Read the model definition and answer for the solid it produces. Units are mm, in the model's axes. Face numbers are marked on the shaded views. A direction names the side the tool comes from. Give positions to 0.01 mm unless a question says otherwise; leave off trailing zeros. Loops run counter-clockwise (first coordinate to the right, second up) from the corner with the lowest first, then second, coordinate; pieces in that order, holes last.
(1) Each of these flat-tipped pins is pushed along its axis until it touches: P1, Ø4, axis at y = 20.5, z = 24.5, coming from the +X side; P2, Ø5, axis at x = 26.5, y = 12, coming from the +Z side; P3, Ø2, axis at x = 18.5, z = 6.5, coming from the +Y side. Where does it stop, or does it pass through?
(2) Determine the mould class of the marked faces 6, 7, 8 and 9 for opening direction Z: pulls with the +Z half, pulls with the -Z half, needs draft (parallel to the pull), parting line crosses it, or undercut.
(3) Which of the six approach directions +Z, -Z, +X, -X, +Y, -Y give full straight-line access (tool end or side, diameter ignored) to the marked faces 1, 2, 3, 4 and 5?
(4) Find section D-D, the plane z = 13. Write down the section's boundary in (x, y), then the cut area to 3 significant figures.
(5) Find section A-A, the plane z = 6. Write down the section's boundary in (x, y), then the cut area to 3 significant figures.
(6) Find section B-B, the plane y = 41.5. Write down the section's boundary in (x, z).
(7) Find section C-C, the plane y = 22.5. Write down the section's boundary in (x, z).
(8) Straight lines are drawn through the part: probe 1 along Y at (x, z) = (19, 9); probe 2 along X at (y, z) = (35, 3.75); probe 3 along Y at (x, z) = (19.2, 12.25). For each, find the intervals that lie inside material, in ascending order.
```python
from build123d import *

# Parameters (mm, degrees)
F1_DEPTH       = 25
F2_W           = 15
F2_H           = 15
F3_DEPTH       = 45
F4_R           = 2
F6_D           = 4
F8_D           = 4
F8_DEPTH       = 15
F8_CSINK_D     = 4.5
F8_CSINK_ANGLE = 90
F8_TIP         = 1.2017212381
F9_R           = 2
F10_DEPTH      = 45
F11_W          = 13.5859974714
F11_H          = 15
F12_DEPTH      = 25.4


with BuildPart() as f1:
    # F0 (on Right) → F1 (new body)
    with BuildSketch(Plane.YZ):
        Polygon((0, 4), (0, 0), (45, 0), (45, 4), (39.5, 4), (39.5, 11), (45, 11), (45, 34), (0, 34), (0, 11), (5.5, 11), (5.5, 4), align=None)
    extrude(amount=F1_DEPTH)

    # F2 (on face) → F3 (cut, through all)
    with BuildSketch(Plane.XZ):
        with Locations((17.5, 26.5)):
            Rectangle(F2_W, F2_H)
    extrude(amount=-F3_DEPTH, mode=Mode.SUBTRACT)

    # F4
    f4_edges = [f1.edges().sort_by_distance(p)[0] for p in [
        (10, 22.5, 34),
        (5, 0, 34),
        (5, 45, 34),
    ]]
    fillet(f4_edges, radius=F4_R)

    # F6 (through all)
    with Locations(Plane(origin=(0, 0, 0), x_dir=(0, -1, 0), z_dir=(-1, 0, 0))):
        with Locations((-22.5, 6)):
            Hole(F6_D / 2)

    # F8
    with Locations(Plane(origin=(0, 0, 0), x_dir=(1, 0, 0), z_dir=(0, 0, -1))):
        with Locations((19.2, -9.6), (6.5, -9.6), (6.5, -35), (19.2, -35)):
            CounterSinkHole(F8_D / 2, F8_CSINK_D / 2, depth=F8_DEPTH, counter_sink_angle=F8_CSINK_ANGLE)
            with Locations((0, 0, -(F8_DEPTH + F8_TIP / 2))):  # 118° drill point
                Cone(0, F8_D / 2, F8_TIP, mode=Mode.SUBTRACT)

    # F9 (on face) → F10 (join, through all)
    with BuildSketch(Plane.XZ):
        with BuildLine():
            Line((32, 19), (25, 19))
            Line((25, 19), (25, 11))
            Line((25, 11), (25.65, 11))
            ThreePointArc((25.65, 11), (30.1401280605, 12.8598719395), (32, 17.35))
            Line((32, 17.35), (32, 19))
        make_face()
        with Locations((28.9811789989, 16.233060509)):
            Circle(F9_R, mode=Mode.SUBTRACT)
    extrude(amount=-F10_DEPTH)

    # F11 (on face) → F12 (cut)
    with BuildSketch(Plane(origin=(0, 0, 0), x_dir=(1, 0, 0), z_dir=(0, 0, -1))):
        with Locations((31.7929987357, -22.5)):
            Rectangle(F11_W, F11_H)
    extrude(amount=-F12_DEPTH, mode=Mode.SUBTRACT)


solid = f1.part
```
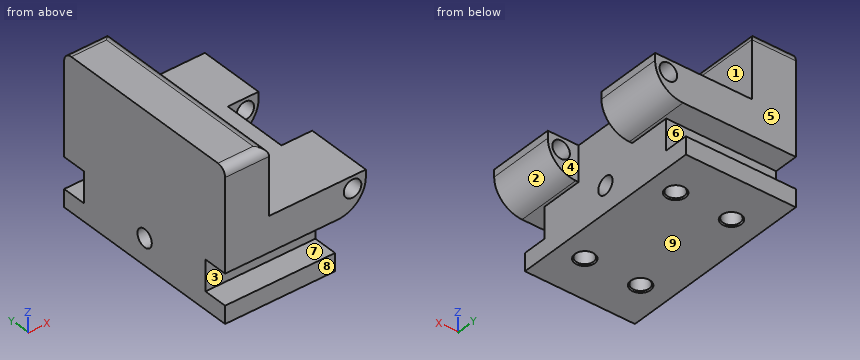
Entries:
1. P1: stops at x = 10
1. P2: stops at z = 19
1. P3: stops at y = 39.5
2. face 6: undercut
2. face 7: undercut
2. face 8: needs draft
2. face 9: pulls with the -Z half
3. face 1: +Z, +X, +Y, -Y
3. face 2: -Z, +X, +Y, -Y
3. face 3: +X, -X, -Y
3. face 4: +Z, -Z, +X
3. face 5: +Z, -Z, +X, -X, +Y
4. outline: (0, 0) - (30.28, 0) - (30.28, 15) - (25, 15) - (25, 30) - (30.28, 30) - (30.28, 45) - (0, 45) - close; hole circle Ø4 at (6.5, 9.6); hole circle Ø4 at (6.5, 35); hole circle Ø4 at (19.2, 9.6); hole circle Ø4 at (19.2, 35)
4. area: 1,230 mm2
5. outline: (0, 5.5) - (25, 5.5) - (25, 20.5) - (0, 20.5) - close; (0, 24.5) - (25, 24.5) - (25, 39.5) - (0, 39.5) - close; hole circle Ø4 at (6.5, 9.6); hole circle Ø4 at (6.5, 35); hole circle Ø4 at (19.2, 9.6); hole circle Ø4 at (19.2, 35)
5. area: 700 mm2
6. outline: (0, 0) - (25, 0) - (25, 4) - (0, 4) - close; (0, 11) - (25.65, 11) arc R6.35 ccw to (32, 17.35) - (32, 19) - (10, 19) - (10, 32) arc R2 ccw to (8, 34) - (0, 34) - close; hole circle Ø4 at (28.98, 16.23)
7. outline: (0, 0) - (25, 0) - (25, 4) - (0, 4) - close; (0, 8) - (25, 8) - (25, 19) - (10, 19) - (10, 32) arc R2 ccw to (8, 34) - (0, 34) - close
8. probe 1: y = 5.5 to 7.61, 11.59 to 33.01, 36.99 to 39.5
8. probe 2: x = 0 to 4.5, 8.5 to 17.2, 21.2 to 25
8. probe 3: y = 0 to 7.6, 11.6 to 33, 37 to 45
